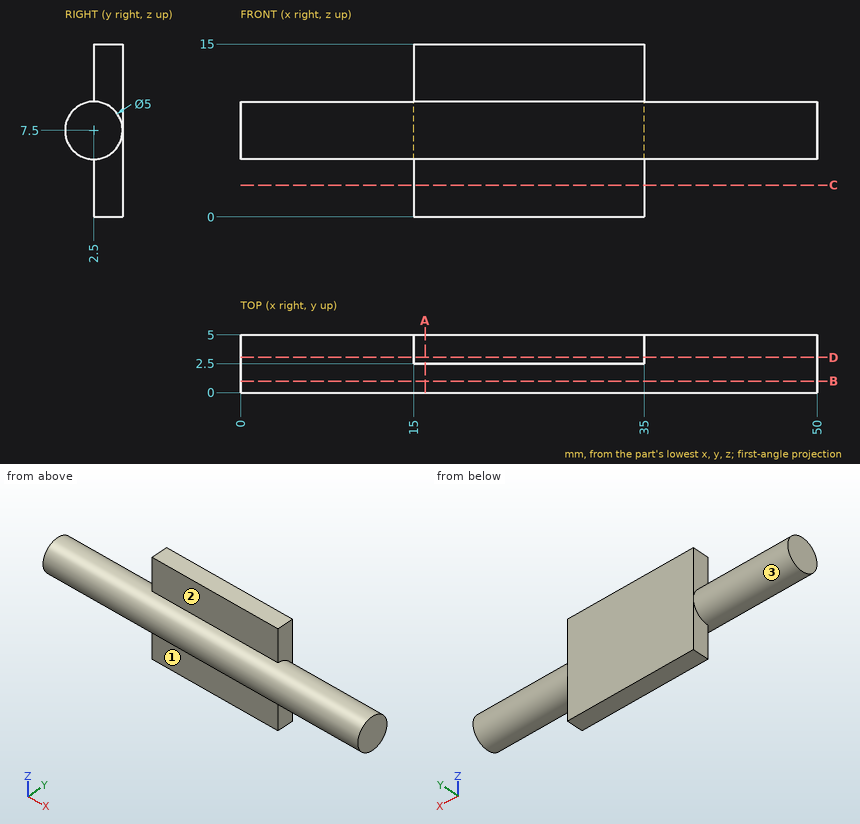
Study the drawing (mm; zero at the part's minimum x, y, z) and answer. A direction names the side the tool comes from. Give positions to 0.01 mm unless a question says otherwise; leave off trailing zeros. Write each loop counter-clockwise with the first axis right and the second up, starting at its lowest first coordinate (ties: lowest second). Pieces come first, ordered by that corner, then holes.
(1) The part is cut by section A-A on x = 16. Write down the section's boundary in (y, z), plus the area to 3 significant figures.
Final values:
outline: (2.5, 0) - (5, 0) - (5, 15) - (2.5, 15) - (2.5, 10) arc R2.5 ccw to (2.5, 5) - close
area: 47.3 mm2
(2) The part is cut by section C-C on z = 2.75. Write down the section's boundary in (x, y), plus the area to 3 significant figures.
Final values:
outline: (15, 2.5) - (35, 2.5) - (35, 5) - (15, 5) - close
area: 50.0 mm2
(3) Which of the six approach directions +Z, -Z, +X, -X, +Y, -Y give full straight-line access (tool end or side, diameter ignored) to the marked faces 1, 2 and 3?
Final values:
face 1: -Z, +X, -X, -Y
face 2: +Z, +X, -X, -Y
face 3: none
(4) Flat-ended cylindrical pins translate along their axes: pin 1 Ø2 at (y, z) = (4, 12) entering from -X; pin 2 Ø8 at (x, z) = (11.5, 2.5) entering from -Y; pin 3 Ø1 at (x, z) = (42, 6) entering from +Y. Find the tip coordinate at first contact, or state that the pin passes through.
Final values:
pin 1: stops at x = 15
pin 2: stops at y = 0.21
pin 3: stops at y = 4.79
(5) The part is cut by section B-B on y = 1. Write down the section's boundary in (x, z), plus the area to 3 significant figures.
Final values:
outline: (0, 5.5) - (50, 5.5) - (50, 9.5) - (0, 9.5) - close
area: 200 mm2
(6) Straight lines are drawn through the part: line 1 (X direction, y = 4.1, z = 11.25); line 2 (Y direction, x = 27.5, z = 14); line 3 (Z direction, x = 23.5, y = 1.2). For each, find the intervals that lie inside material, in ascending order.
Final values:
line 1: x = 15 to 35
line 2: y = 2.5 to 5
line 3: z = 5.36 to 9.64
(7) The part is cut by section D-D on y = 3.05. Write down the section's boundary in (x, z), plus the area to 3 significant figures.
Final values:
outline: (0, 5.06) - (15, 5.06) - (15, 0) - (35, 0) - (35, 5.06) - (50, 5.06) - (50, 9.94) - (35, 9.94) - (35, 15) - (15, 15) - (15, 9.94) - (0, 9.94) - close
area: 446 mm2
